Autodesk Inventor part; units mm, degrees
ref_plane "YZ Plane" through (0, 0, 0) normal (1, 0, 0) x (0, 1, 0)
ref_plane "XZ Plane" through (0, 0, 0) normal (0, 1, 0) x (-1, 0, 0)
ref_plane "XY Plane" through (0, 0, 0) normal (0, 0, 1) x (1, 0, 0)
sketch "スケッチ1" plane through (0, 0, 0) normal (0, 0, 1) x (1, 0, 0)
  arc A0 (69.7697, -24.216) -> (68.6872, -22.341) centre (68.6872, -23.591) ccw
  arc A1 (69.7697, -24.216) -> (69.7697, -25.716) centre (71.0687, -24.966) ccw
  arc A2 (68.6872, -27.591) -> (69.7697, -25.716) centre (68.6872, -26.341) ccw
  arc A3 (65.2231, -28.341) -> (67.3881, -28.341) centre (66.3056, -27.716) ccw
  arc A4 (68.6872, -27.591) -> (67.3881, -28.341) centre (68.6872, -29.091) ccw
  arc A5 (65.2231, -28.341) -> (63.924, -27.591) centre (63.924, -29.091) ccw
  arc A6 (63.924, -22.341) -> (62.8415, -24.216) centre (63.924, -23.591) ccw
  arc A7 (63.924, -22.341) -> (65.2231, -21.591) centre (63.924, -20.841) ccw
  line L0 (62.8415, -22.966) -> (66.3056, -20.966) construction
  circle A8 centre (66.3056, -24.966) radius 5
  arc A9 (67.3881, -21.591) -> (65.2231, -21.591) centre (66.3056, -22.216) ccw
  arc A10 (62.8415, -25.716) -> (62.8415, -24.216) centre (61.5425, -24.966) ccw
  arc A11 (67.3881, -21.591) -> (68.6872, -22.341) centre (68.6872, -20.841) ccw
  line L1 (62.8415, -26.966) -> (62.8415, -22.966) construction
  arc A12 (62.8415, -25.716) -> (63.924, -27.591) centre (63.924, -26.341) ccw
  line L2 (66.3056, -20.966) -> (69.7697, -22.966) construction
  line L3 (66.3056, -28.966) -> (62.8415, -26.966) construction
  circle A13 centre (66.3056, -24.966) radius 4 construction
  circle A14 centre (66.3056, -24.966) radius 3.2631 construction
  line L4 (69.7697, -26.966) -> (66.3056, -28.966) construction
  line L5 (69.7697, -22.966) -> (69.7697, -26.966) construction
  circle A15 centre (66.3056, -24.966) radius 2.025
  point P0 (0, 0)
  point P1 (69.7697, -26.966)
  point P2 (66.3056, -28.966)
  point P3 (65.2231, -28.341)
  point P4 (68.6872, -27.591)
  point P5 (69.7697, -25.716)
  point P6 (69.7697, -24.216)
  point P7 (63.924, -22.341)
  point P8 (62.8415, -25.716)
  point P9 (63.924, -27.591)
  dimension "d5" = 8
  dimension "d4" = 10
  dimension "d6" = 360
  dimension "d7" = 360
  dimension "d8" = 6.5263
  dimension "d9" = 1.5
  dimension "d10" = 1.25
  dimension "d11" = 4.05
extrude "押し出し1" add sketch "スケッチ1" along normal blind 4.5 contours A1 A2 A4 A3 A5 A12 A10 A6 A7 A9 A11 A0
sketch "スケッチ2" plane through (0, 0, 4.5) normal (0, 0, 1) x (1, 0, 0)
  arc A0 (68.6872, -27.591) -> (67.3881, -28.341) centre (68.6872, -29.091) ccw
  arc A1 (68.6872, -27.591) -> (69.7697, -25.716) centre (68.6872, -26.341) ccw
  arc A2 (69.7697, -24.216) -> (69.7697, -25.716) centre (71.0687, -24.966) ccw
  arc A3 (69.7697, -24.216) -> (68.6872, -22.341) centre (68.6872, -23.591) ccw
  arc A4 (67.3881, -21.591) -> (68.6872, -22.341) centre (68.6872, -20.841) ccw
  arc A5 (67.3881, -21.591) -> (65.2231, -21.591) centre (66.3056, -22.216) ccw
  arc A6 (63.924, -22.341) -> (65.2231, -21.591) centre (63.924, -20.841) ccw
  arc A7 (63.924, -22.341) -> (62.8415, -24.216) centre (63.924, -23.591) ccw
  arc A8 (62.8415, -25.716) -> (62.8415, -24.216) centre (61.5425, -24.966) ccw
  arc A9 (62.8415, -25.716) -> (63.924, -27.591) centre (63.924, -26.341) ccw
  arc A10 (65.2231, -28.341) -> (63.924, -27.591) centre (63.924, -29.091) ccw
  arc A11 (65.2231, -28.341) -> (67.3881, -28.341) centre (66.3056, -27.716) ccw
  circle A12 centre (66.3056, -24.966) radius 2.025
  circle A13 centre (66.3056, -24.966) radius 5
  point P0 (0, 0)
  dimension "d14" = 10
extrude "押し出し2" add sketch "スケッチ2" along normal blind 0.8 contours A0 A11 A10 A9 A8 A7 A6 A5 A4 A3 A2 A1 | A13
sketch "スケッチ3" plane through (0, 0, 0) normal (0, 0, -1) x (-1, 0, 0)
  arc A0 (-67.3881, -28.341) -> (-68.6872, -27.591) centre (-68.6872, -29.091) ccw
  arc A1 (-67.3881, -28.341) -> (-65.2231, -28.341) centre (-66.3056, -27.716) ccw
  arc A2 (-63.924, -27.591) -> (-65.2231, -28.341) centre (-63.924, -29.091) ccw
  arc A3 (-63.924, -27.591) -> (-62.8415, -25.716) centre (-63.924, -26.341) ccw
  arc A4 (-62.8415, -24.216) -> (-62.8415, -25.716) centre (-61.5425, -24.966) ccw
  arc A5 (-62.8415, -24.216) -> (-63.924, -22.341) centre (-63.924, -23.591) ccw
  arc A6 (-65.2231, -21.591) -> (-63.924, -22.341) centre (-63.924, -20.841) ccw
  arc A7 (-65.2231, -21.591) -> (-67.3881, -21.591) centre (-66.3056, -22.216) ccw
  arc A8 (-68.6872, -22.341) -> (-67.3881, -21.591) centre (-68.6872, -20.841) ccw
  arc A9 (-68.6872, -22.341) -> (-69.7697, -24.216) centre (-68.6872, -23.591) ccw
  arc A10 (-69.7697, -25.716) -> (-69.7697, -24.216) centre (-71.0687, -24.966) ccw
  arc A11 (-69.7697, -25.716) -> (-68.6872, -27.591) centre (-68.6872, -26.341) ccw
  circle A12 centre (-66.3056, -24.966) radius 2.025
  arc A13 (-65.2664, -21.616) -> (-67.3448, -21.616) centre (-66.3056, -22.216) ccw
  arc A14 (-65.2664, -21.616) -> (-63.924, -22.391) centre (-63.924, -20.841) ccw
  arc A15 (-62.8848, -24.191) -> (-63.924, -22.391) centre (-63.924, -23.591) ccw
  arc A16 (-62.8848, -24.191) -> (-62.8848, -25.741) centre (-61.5425, -24.966) ccw
  arc A17 (-63.924, -27.541) -> (-62.8848, -25.741) centre (-63.924, -26.341) ccw
  arc A18 (-63.924, -27.541) -> (-65.2664, -28.316) centre (-63.924, -29.091) ccw
  arc A19 (-67.3448, -28.316) -> (-65.2664, -28.316) centre (-66.3056, -27.716) ccw
  arc A20 (-67.3448, -28.316) -> (-68.6872, -27.541) centre (-68.6872, -29.091) ccw
  arc A21 (-69.7264, -25.741) -> (-68.6872, -27.541) centre (-68.6872, -26.341) ccw
  arc A22 (-69.7264, -25.741) -> (-69.7264, -24.191) centre (-71.0687, -24.966) ccw
  arc A23 (-68.6872, -22.391) -> (-69.7264, -24.191) centre (-68.6872, -23.591) ccw
  arc A24 (-68.6872, -22.391) -> (-67.3448, -21.616) centre (-68.6872, -20.841) ccw
  point P0 (0, 0)
  dimension "d17" = 0.05
extrude "押し出し3" cut sketch "スケッチ3" against normal up to surface (4.5 mm away) contours A0 A11 A10 A9 A8 A7 A6 A5 A4 A3 A2 A1
properties part number "2ギア接続部" material "アルミニウム 2014-T4"
Source: CAD feature listing. Evaluate the final solid. Frame: model axes, mm. A direction names the side the tool comes from. Coordinates: 2 decimals unless noted, no trailing zeros. Order: outer loops, then holes, each group sorted by start corner. A loop starts at its lowest first (then second) coordinate and runs counter-clockwise, first axis right, second up. Notation, with made-up numbers: M 80,56.25 L 136,56.25 A10 ccw 136,72.25 Z; hole C 55.25,9.5 d1. An arc over 180 degrees is marked long. Write each question's results on one line, items separated by ' | '. Start each with the question number.
1) Contact query for a flat-ended pin moving along its axis: pin 1 Ø1 at (x, y) = (66, -28.5) entering from -Z. Output: stop coordinate, or through.
2) Line query: line 1 (Z direction, x = 68.5, y = -29); line 2 (Y direction, x = 68.75, z = 3.55); line 3 (X direction, y = -24.75, z = 3.2). Output: solid intervals per line, ascending. Write a range as from..to.
3) Section query D-D (x = 63.5). Return the cut outline in (y, z), plus the area to 3 significant figures.
4) Access query for faces 1 (the face through (66.323, -28.916, 2.218)), 2 (the face through (63.092, -24.955, 2.218)), 3 (the face through (69.72, -22.98, 2.22)). Directions: +Z, -Z, +X, -X, +Y, -Y. A direction counts if a zero-diameter tool reaches every point of the face in a straight line with its end or side. Return the directions, or none.
5) Draft query along X for faces 4 (the face through (66.288, -21.016, 2.218)), 5 (the face through (69, -25, 0)), 6 (the face through (64.283, -25.055, 2.613)). Return one class per face: released by +X, released by -X, zero draft, split by the parting line, or undercut.
6) Section query A-A (y = -26). Return the cut outline in (x, z), plus the area to 3 significant figures.
7) Section query B-B (x = 66.75). Return the cut outline in (y, z).
Answers:
1) pin 1: stops at z = 0
2) line 1: z = 4.5..5.3 | line 2: y = -27.54..-22.39 | line 3: x = 63.08..64.29, 68.32..69.53
3) outline: M -29.1,4.5 L -27.46,4.5 L -27.46,0 L -22.47,0 L -22.47,4.5 L -20.83,4.5 L -20.83,5.3 L -29.1,5.3 Z | area: 29.1 mm^2
4) face 1: -Z, -Y | face 2: -Z, -X | face 3: -Z, +X
5) face 4: split by the parting line | face 5: zero draft | face 6: undercut
6) outline: M 61.41,4.5 L 62.77,4.5 L 62.77,0 L 64.56,0 L 64.56,5.3 L 61.41,5.3 Z; M 68.05,0 L 69.84,0 L 69.84,4.5 L 71.2,4.5 L 71.2,5.3 L 68.05,5.3 Z | area: 21.2 mm^2
7) outline: M -29.95,4.5 L -28.83,4.5 L -28.83,0 L -26.94,0 L -26.94,5.3 L -29.95,5.3 Z; M -22.99,0 L -21.1,0 L -21.1,4.5 L -19.99,4.5 L -19.99,5.3 L -22.99,5.3 Z
